Check sheet for the modelled part. Datum: model origin and axes. Units: mm. Round coordinates to 2 decimals unless told otherwise and drop trailing zeros. Write each loop counter-clockwise with the first axis right and the second up, starting at its lowest first coordinate (ties: lowest second). Pieces come first, ordered by that corner, then holes. Notation, with made-up numbers: (-35.75, 47) - (-18.75, 47) arc R18 ccw to (-18.75, 56) - close; hole circle Ø7 at (15, 25.5). An arc over 180 degrees is marked (long way). Use one line per item in the form item = value. Start each with the question number.
1) Draft check along X on faces 1 (the face through (0.873, 32.772, 2.344)), 2 (the face through (17.594, 35.219, 3.944)), 3 (the face through (-27.719, 35.094, 3.944)). Enter one of: +X half, -X half, draft (parallel to the pull), parting line (faces both ways), or undercut.
2) Section check B-B (x = 0). Record the boundary of the cut face in (y, z), then the cut area to 4 significant figures.
3) Section check C-C (x = -20). Record the boundary of the cut face in (y, z), then the cut area to 4 significant figures.
4) Gauge pin test, flat ends, axial feed: P1, Ø4, axis at x = 9.9, y = 11.9, coming from the +Z side; P2, Ø9, axis at x = -20, y = -30, coming from the -Z side. Record the tip position at first contact, or that the pin passes through.
5) Section check A-A (y = 2). Record the boundary of the cut face in (x, z), then the cut area to 3 significant figures.
6) Scan lines: probe 1 along Y at (x, z) = (0, 6.9); probe 2 along X at (y, z) = (30, 6.6); probe 3 along Y at (x, z) = (2, 6.5). Record each from-to range of solid material in increasing order.
7) Section check D-D (z = 1.75). Count the separate pieces of the cut face and the enclosed holes in it, then the cut area to 3 significant figures.
Autodesk Inventor part; units mm, degrees
ref_plane "YZ Plane" through (0, 0, 0) normal (1, 0, 0) x (0, 1, 0)
ref_plane "XZ Plane" through (0, 0, 0) normal (0, 1, 0) x (-1, 0, 0)
ref_plane "XY Plane" through (0, 0, 0) normal (0, 0, 1) x (1, 0, 0)
sketch "Эскиз1" plane through (0, 0, 0) normal (0, 0, 1) x (1, 0, 0)
  line L0 (-1.5933, 37.5) -> (12, 37.5)
  line L1 (20, 29.5) -> (20, -29.5)
  arc A0 (20, 29.5) -> (12, 37.5) centre (12, 29.5) ccw
  line L2 (-1.5933, 37.5) -> (-22, 37.5)
  line L3 (-30, 29.5) -> (-30, -29.5)
  arc A1 (-22, 37.5) -> (-30, 29.5) centre (-22, 29.5) ccw
  line L4 (-42.3196, 0) -> (32.3196, 0)
  line L5 (0, -54.8196) -> (0, 54.8196)
  circle A2 centre (0, 2) radius 11.25
  circle A3 centre (0, 2) radius 14 construction
  line L6 (0, 2) -> (-9.8995, 11.8995) construction
  line L7 (-22, -37.5) -> (12, -37.5)
  arc A4 (-30, -29.5) -> (-22, -37.5) centre (-22, -29.5) ccw
  arc A5 (12, -37.5) -> (20, -29.5) centre (12, -29.5) ccw
  line L8 (0, 30) -> (-20, 30) construction
  line L9 (0, -30) -> (-20, -30) construction
  point P0 (0, 0)
  point P1 (0, 0)
  point P2 (0, 54.8196)
  point P3 (9.8995, 11.8995)
  point P4 (-9.8995, -7.8995)
  point P5 (9.8995, -7.8995)
  point P6 (20, 0)
  dimension "d128" = 28
  dimension "d43" = 8
  dimension "d50" = 20
  dimension "d127" = 22.5
  dimension "d131" = 360
  dimension "d134" = 45
  dimension "d168" = 7.5
  dimension "d182" = 2
  dimension "d200" = 20
  dimension "d201" = 50
  dimension "d202" = 75
extrude "Пластина2" add sketch "Эскиз1" along normal blind 8 contours L0 L5 A2 L4 L3 A1 L2 | L0 A0 L1 L4 A2 L5 | A2 L5 L7 A4 L3 L4 | L1 A5 L7 L5 A2 L4
hole "Отверстие2" at (-20, 30, 0) at (0, 30, 0) at (0, -30, 0) at (-20, -30, 0) direction (0, 0, 1) diameter 5.5 end through all countersink diameter 10.5 countersink angle 90
sketch "Эскиз6" plane through (0, 0, 8) normal (0, 0, 1) x (1, 0, 0)
  circle A0 centre (0, 2) radius 14 construction
  line L0 (0, -54.8196) -> (0, 54.8196)
  line L1 (-42.3196, 0) -> (32.3196, 0)
  line L2 (0, 2) -> (9.8995, 11.8995) construction
  point P0 (-9.8995, 11.8995)
  point P1 (-9.8995, -7.8995)
  point P2 (9.8995, -7.8995)
  dimension "d135" = 28
  dimension "d138" = 360
  dimension "d141" = 135
  dimension "d183" = 2
hole "Отверстие3" at (-9.8995, -7.8995, 8) at (9.8995, 11.8995, 8) at (-9.8995, 11.8995, 8) at (9.8995, -7.8995, 8) direction (0, 0, -1) diameter 4.5 end through all
equation "\"d18\" = Толщина"
equation "\"Радиус_гибки\" = Толщина"
equation "\"Ширина_просечки\" = Толщина"
equation "\"Глубина_просечки\" = 0.5 * Толщина"
equation "\"Размер_просечки\" = 4 * Толщина"
equation "\"Мин_остаток\" = 2 * Толщина"
equation "\"Радиус_перехода\" = Радиус_гибки"
equation "\"Радиус_Якоби\" = Радиус_гибки"
equation "\"Размер_зазора\" = Толщина"
properties part number "кронштейн" material "Сталь"
Results are:
q1.face_1 = undercut
q1.face_2 = +X half
q1.face_3 = -X half
q2.outline = (-37.5, 0) - (-35.25, 0) - (-32.75, 2.5) - (-32.75, 8) - (-37.5, 8) - close; (-27.25, 2.5) - (-24.75, 0) - (-9.25, 0) - (-9.25, 8) - (-27.25, 8) - close; (13.25, 0) - (24.75, 0) - (27.25, 2.5) - (27.25, 8) - (13.25, 8) - close; (32.75, 2.5) - (35.25, 0) - (37.5, 0) - (37.5, 8) - (32.75, 8) - close
q2.area = 319.5 mm²
q3.outline = (-37.5, 0) - (-35.25, 0) - (-32.75, 2.5) - (-32.75, 8) - (-37.5, 8) - close; (-27.25, 2.5) - (-24.75, 0) - (24.75, 0) - (27.25, 2.5) - (27.25, 8) - (-27.25, 8) - close; (32.75, 2.5) - (35.25, 0) - (37.5, 0) - (37.5, 8) - (32.75, 8) - close
q3.area = 499.5 mm²
q4.P1 = through
q4.P2 = 0.75
q5.outline = (-30, 0) - (-11.25, 0) - (-11.25, 8) - (-30, 8) - close; (11.25, 0) - (20, 0) - (20, 8) - (11.25, 8) - close
q5.area = 220 mm²
q6.probe_1 = -37.5 to -32.75, -27.25 to -9.25, 13.25 to 27.25, 32.75 to 37.5
q6.probe_2 = -29.98 to -22.75, -17.25 to -2.75, 2.75 to 19.98
q6.probe_3 = -37.5 to -31.89, -28.11 to -9.07, 13.07 to 28.11, 31.89 to 37.5
q7.separate_pieces = 1
q7.enclosed_holes = 9
q7.area = 3,080 mm²
